Source: three-view drawing plus pictorial views. Frame: mm from the lowest corner of the part. Give positions to 0.01 mm unless a question says otherwise; leave off trailing zeros. Loops run counter-clockwise (first coordinate to the right, second up) from the corner with the lowest first, then second, coordinate; pieces in that order, holes last. Notation, with made-up numbers: M -13,2 L 44,2 A17 ccw 44,13 Z; hole C 83,19 d4. An arc over 180 degrees is marked long. Put each result on its own line as item: value. Start each with the question number.
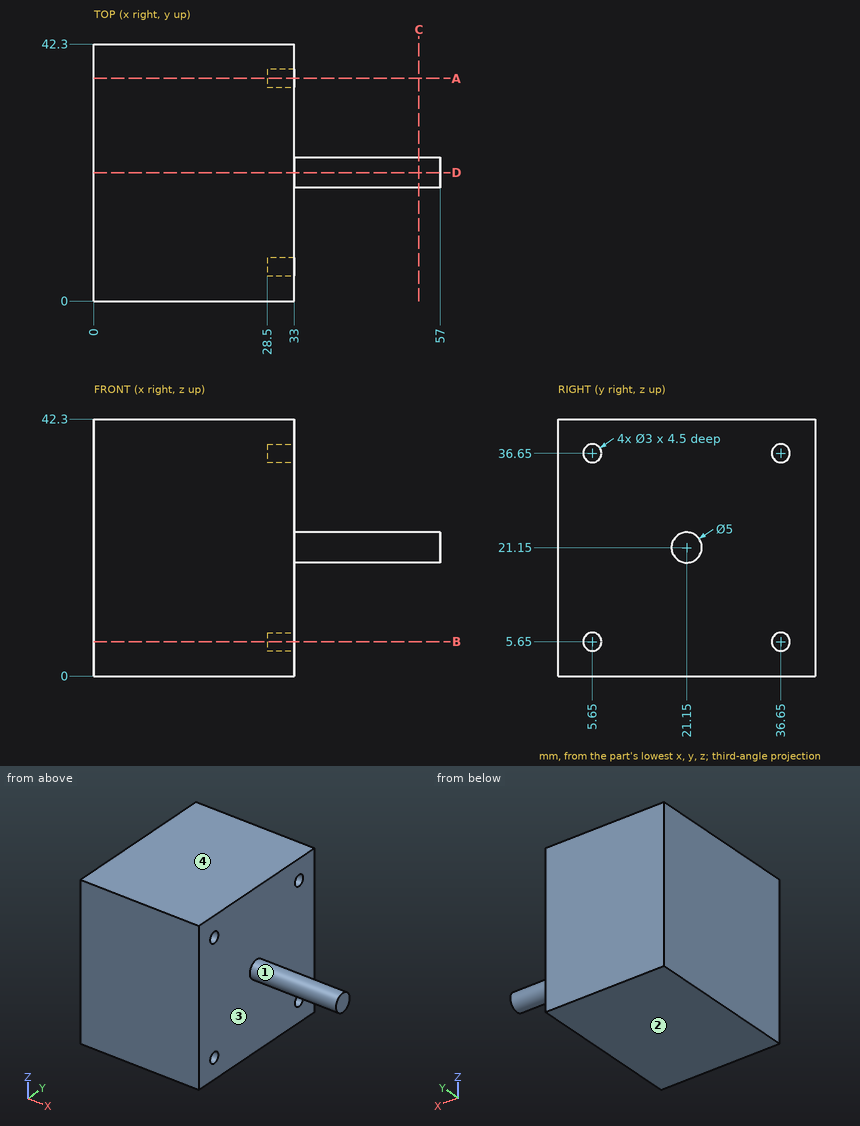
1. Section A-A, the plane y = 36.65. Output: boundary loops of the cut face in (x, z).
2. Pull-direction query (Z, two-part tool) for the marked faces 1, 2, 3 and 4; classes: released by +Z, released by -Z, zero draft, split by the parting line, or undercut.
3. Contact query for flat-ended pins moving along their axis: pin 1 (2.5 mm diameter, centred on y = 36.65, z = 5.65, fed in from +X); pin 2 (8 mm diameter, centred on y = 12.5, z = 16, fed in from +X); pin 3 (1 mm diameter, centred on x = 34, z = 20.5, fed in from +Y). Output: stop coordinate, or through.
4. Section C-C, the plane x = 53.5. Output: boundary loops of the cut face in (y, z), plus the area to 3 significant figures.
5. Ray query, line 1 (Z direction, x = 29.6, y = 5.65); line 2 (Y direction, x = 31, z = 36). Return the intervals inside material, ascending.
6. Section D-D, the plane y = 21.15. Output: boundary loops of the cut face in (x, z).
Results found:
1. outline: M 0,0 L 33,0 L 33,4.15 L 28.5,4.15 L 28.5,7.15 L 33,7.15 L 33,35.15 L 28.5,35.15 L 28.5,38.15 L 33,38.15 L 33,42.3 L 0,42.3 Z
2. face 1: split by the parting line
2. face 2: released by -Z
2. face 3: zero draft
2. face 4: released by +Z
3. pin 1: x = 28.5
3. pin 2: x = 33
3. pin 3: y = 23.65
4. outline: C 21.15,21.15 d5
4. area: 19.6 mm²
5. line 1: 0 to 4.15, 7.15 to 35.15, 38.15 to 42.3
5. line 2: 0 to 4.3, 7 to 35.3, 38 to 42.3
6. outline: M 0,0 L 33,0 L 33,18.65 L 57,18.65 L 57,23.65 L 33,23.65 L 33,42.3 L 0,42.3 Z
